Autodesk Inventor part; units mm, degrees
ref_plane "YZ Plane" through (0, 0, 0) normal (1, 0, 0) x (0, 1, 0)
ref_plane "XZ Plane" through (0, 0, 0) normal (0, 1, 0) x (-1, 0, 0)
ref_plane "XY Plane" through (0, 0, 0) normal (0, 0, 1) x (1, 0, 0)
sketch "Sketch1" plane through (0, 0, 0) normal (0, 0, 1) x (1, 0, 0)
  line L0 (0, 0) -> (236.4232, 0)
  line L1 (236.4232, 0) -> (236.4232, -176.7078)
  line L2 (236.4232, -176.7078) -> (0, -176.7078)
  line L3 (0, -176.7078) -> (0, 0)
  dimension "d0" = 236.4232
  dimension "d1" = 176.7078
extrude "Extrusion1" add sketch "Sketch1" along normal blind 3.81
chamfer "Chamfer1" distance 38.1 angle 45 1 edges at (236.4232, 0, 1.905)
chamfer "Chamfer2" distance 38.1 angle 45 1 edges at (0, 0, 1.905)
chamfer "Chamfer3" distance 38.1 angle 45 1 edges at (236.4232, -176.7078, 1.905)
chamfer "Chamfer4" distance 38.1 angle 45 1 edges at (0, -176.7078, 1.905)
move faces "Move1" translate (0, 22.098, 0) faces at (91.5077, 0, 1.27)
sketch "Sketch2" plane through (198.3232, -176.7078, 0) normal (0, -1, 0) x (1, 0, 0)
  point P0 (-198.3232, 0)
properties part number "ElectronicsPlate2"
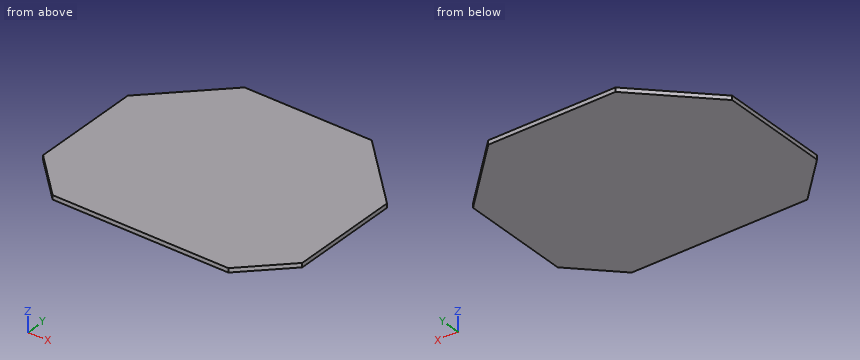
Model file for the job. Use its own axes, mm. Coordinates: 2 decimals unless noted, no trailing zeros. Write each loop counter-clockwise with the first axis right and the second up, starting at its lowest first coordinate (ties: lowest second). Pieces come first, ordered by that corner, then holes. Notation, with made-up numbers: (88, 18) - (119, 18) arc R23 cw to (119, 37) - close; hole circle Ø6 at (27.25, -13.5). An arc over 180 degrees is marked (long way). Use a Markdown table: item, result. Add a question column.
Item 1: Band-saw the part on B-B, the plane x = 205.5. Write the cut outline in (y, z).
Item 2: Band-saw the part on C-C, the plane y = -154. Write the cut outline in (x, z), and give its area (3 significant figures).
Item 3: Drill centre lines: line 1 along X through (y, z) = (0, 2.4); line 2 along X through (y, z) = (2, 0.75); line 3 along Y through (x, z) = (223, 2.7). Where is each one in solid material? Low to high.
Item 4: Band-saw the part on A-A, the plane z = 3.1. Write the cut outline in (x, y).
Item 5: Drop a flat-ended pin along its axis: pin 1 (6 mm diameter, centred on x = 200.5, y = -95, fed in from -Z). Give the stop position or say it passes through.
A:
| question | item | result |
|---|---|---|
| 1 | outline | (-169.53, 0) - (-7.18, 0) - (-7.18, 3.81) - (-169.53, 3.81) - close |
| 2 | outline | (15.39, 0) - (221.03, 0) - (221.03, 3.81) - (15.39, 3.81) - close |
| 2 | area | 783 mm² |
| 3 | line 1 | x = 38.1 to 198.32 |
| 3 | line 2 | x = 40.1 to 196.32 |
| 3 | line 3 | y = -152.03 to -24.68 |
| 4 | outline | (0, -138.61) - (38.1, -176.71) - (198.32, -176.71) - (236.42, -138.61) - (236.42, -38.1) - (176.23, 22.1) - (60.2, 22.1) - (0, -38.1) - close |
| 5 | pin 1 | stops at z = 0 |
